Source: CAD feature listing. Evaluate the final solid. Frame: model axes, mm. A direction names the side the tool comes from. Give positions to 0.01 mm unless a question says otherwise; leave off trailing zeros. Write each loop counter-clockwise with the first axis right and the second up, starting at its lowest first coordinate (ties: lowest second). Pieces come first, ordered by that corner, then holes. Notation, with made-up numbers: (-39.5, -27.75) - (-11.5, -27.75) arc R18 cw to (-11.5, -4.75) - close; hole circle Ø1 at (62, 1). An arc over 180 degrees is marked (long way). Answer as a JSON object with one key per item and string values. Group by question number.
from build123d import *

# Parameters (mm, degrees)
SKETCH001_R       = 0.95
PAD001_DEPTH      = 13.08
PAD001_DEPTH_BACK = 3.5
SKETCH_R          = 20.32
SKETCH_R_2        = 2.225
PAD_DEPTH         = 26.16
FILLET_R          = 0.5


with BuildPart() as pad001:
    # Sketch001 → Pad001 (new body, two sides)
    with BuildSketch(Plane.XY.offset(0.5)) as pad001_sk:
        Circle(SKETCH001_R)
        with Locations((27.94, 0)):
            Circle(SKETCH001_R)
    extrude(amount=PAD001_DEPTH)
    extrude(pad001_sk.sketch, amount=-PAD001_DEPTH_BACK)


with BuildPart() as obj1:
    # Sketch → Pad (new body)
    with BuildSketch(Plane.XY.offset(0.1)):
        with Locations((13.97, 0)):
            Circle(SKETCH_R)
        with Locations((13.97, 0)):
            Circle(SKETCH_R_2, mode=Mode.SUBTRACT)
    extrude(amount=PAD_DEPTH)

    # Fillet
    fillet_edges = [obj1.edges().sort_by_distance(p)[0] for p in [
        (11.745, 0, 26.26),
        (-6.35, 0, 26.26),
        (-6.35, 0, 0.1),
    ]]
    fillet(fillet_edges, radius=FILLET_R)

    # obj1: union Pad001
    add(pad001.part)


solid = obj1.part
Q1. First-contact query: pin 1 Ø4 at (x, y) = (2.5, 13.5) entering from -Z; pin 2 Ø5 at (y, z) = (-4, 4.5) entering from -X; pin 3 Ø4 at (x, z) = (24, 17.5) entering from +Y. Flat tips, straight axial feed; report the tip coordinate or a pass-through.
Q2. Section B-B on x = 13.97. Return the cut outline in (y, z) (3 decimals).
Q3. Ray query, probe 1 along Y at (x, z) = (13.97, 13.75) (3 decimals); probe 2 along Z at (x, y) = (11, -5); probe 3 along X at (y, z) = (-1, 21). Return the intervals inside material, ascending. Write a range as [from, to].
Q4. Draft query along X for faces 1 (the cylindrical face through (33.352, 6.104, 13.004)), 2 (the cylindrical face through (-0.95, 0.04, -1.43)), 3 (the flat face through (28, 0, -3)). Return one class per face: released by +X, released by -X, zero draft, split by the parting line, or undercut.
Q5. Reachability of faces 4 (the cylindrical face through (12.2, -1.35, 12.75)), 5 (the cylindrical face through (28.846, 0.285, -1.428)) from +Z, -Z, +X, -X, +Y, -Y: full face, straight path, thin tool, end or side. Return the list, or none.
Q6. Section C-C on z = 21.25. Return the cut outline in (x, y) (3 decimals).
Q7. Section A-A on y = 0. Return the cut outline in (x, z) (3 decimals), then the cut area to 3 significant figures.
Taken from the geometry:
{
 "1": {"pin 1": "stops at z = 0.1", "pin 2": "stops at x = -6.29", "pin 3": "stops at y = 18.67"},
 "2": {"outline": "(-20.32, 0.6) arc R0.5 ccw to (-19.82, 0.1) - (-2.225, 0.1) - (-2.225, 25.76) arc R0.5 ccw to (-2.725, 26.26) - (-19.82, 26.26) arc R0.5 ccw to (-20.32, 25.76) - close; (2.225, 0.1) - (19.82, 0.1) arc R0.5 ccw to (20.32, 0.6) - (20.32, 25.76) arc R0.5 ccw to (19.82, 26.26) - (2.725, 26.26) arc R0.5 ccw to (2.225, 25.76) - close"},
 "3": {"probe 1": "y = [-20.32, -2.225], [2.225, 20.32]", "probe 2": "z = [0.1, 26.26]", "probe 3": "x = [-6.33, 11.98], [15.96, 34.27]"},
 "4": {"face 1": "split by the parting line", "face 2": "undercut", "face 3": "zero draft"},
 "5": {"face 4": "+Z, -Z", "face 5": "-Z"},
 "6": {"outline": "circle Ø40.64 at (13.97, 0); hole circle Ø4.45 at (13.97, 0)"},
 "7": {"outline": "(-6.35, 0.6) arc R0.5 ccw to (-5.85, 0.1) - (-0.95, 0.1) - (-0.95, -3) - (0.95, -3) - (0.95, 0.1) - (11.745, 0.1) - (11.745, 25.76) arc R0.5 ccw to (11.245, 26.26) - (-5.85, 26.26) arc R0.5 ccw to (-6.35, 25.76) - close; (16.195, 0.1) - (26.99, 0.1) - (26.99, -3) - (28.89, -3) - (28.89, 0.1) - (33.79, 0.1) arc R0.5 ccw to (34.29, 0.6) - (34.29, 25.76) arc R0.5 ccw to (33.79, 26.26) - (16.695, 26.26) arc R0.5 ccw to (16.195, 25.76) - close", "area": "958 mm²"}
}
